Can you work these out from the model? Positions are in its coordinate system, mm. A direction names the side the tool comes from. Give positions to 0.01 mm unless a question says otherwise; leave off trailing zeros. Loops run counter-clockwise (first coordinate to the right, second up) from the corner with the lowest first, then second, coordinate; pieces in that order, holes last. Notation, with made-up numbers: M 41.25,70.5 L 71.25,70.5 A20 cw 71.25,93.5 Z; hole C 50.5,-27 d7. An arc over 180 degrees is marked long. One line per item, written item: value. Start each with the question number.
Solid Edge part; units mm, degrees
sketch "Sketch1" plane through (0, 0, 0) normal (0, 0, 1) x (1, 0, 0)
  circle A0 centre (-86, 0) radius 8
  circle A1 centre (-43, -74.4782) radius 8
  circle A2 centre (43, -74.4782) radius 8
  circle A3 centre (86, 0) radius 8
  circle A4 centre (43, 74.4782) radius 8
  circle A5 centre (-43, 74.4782) radius 8
  circle A6 centre (0, 0) radius 101.5
extrude "Protrusion1" add sketch "Sketch1" along normal blind 19
sketch "Sketch2" plane through (0, 0, 19) normal (0, 0, 1) x (0, 1, 0)
  circle A0 centre (0, 0) radius 32
  circle A1 centre (0, 0) radius 16
extrude "ExtrudedProtrusion_4" add sketch "Sketch2" along normal blind 51
sketch "Sketch3" plane through (0, 0, 0) normal (1, 0, 0) x (0, 1, 0)
  line L0 (-101.5, 19) -> (-32, 70)
  line L1 (-32, 70) -> (-30, 70)
  line L2 (-30, 70) -> (-30, 19)
  line L3 (-30, 19) -> (-101.5, 19)
extrude "ExtrudedCutout_5" cut sketch "Sketch3" along normal mid plane 16
sketch "Sketch4" plane through (0, 0, 0) normal (1, 0, 0) x (0, 1, 0)
  line L0 (-101.5, 19) -> (-32, 70)
  line L1 (-32, 70) -> (-30, 70)
  line L2 (-30, 70) -> (-30, 19)
  line L3 (-30, 19) -> (-101.5, 19)
extrude "ExtrudedProtrusion_9" add sketch "Sketch4" along normal mid plane 16
pattern_circular "Pattern1" count 3 over 360 about axis through (0, 0, 70) along (0, 0, 1) of "ExtrudedProtrusion_9"
Q1. If we section it at B-B, the plane x = -43: Write out the boundary of the cut face in (y, z).
Q2. For P1, Ø21, axis at x = -86, y = 0, coming from the +Z side; P2, Ø5, axis at x = 6, y = -47, coming from the -Z side; P3, Ø14.5, axis at x = 43, y = -74.48, coming from the +Z side; P4, Ø10, axis at x = -28, z = 44, coming from the +Y side, each with a flat end and sliding along its axis, tell me the tip position at first contact or that it passes through.
Q3. If we section it at C-C, the plane z = 39: Write out the boundary of the cut face in (x, y).
Q4. If we mould it in two halves opening along X, with no side actions, what happens to faces 1 (the face through (-48.9, -79.88, 9.37)), 2 (the face through (96.813, -30.488, 9.367)), 3 (the face through (-8, -51, 34))? For each: released by +X, released by -X, zero draft, split by the parting line, or undercut.
Q5. If we section it at A-A, the plane y = 0: Write out the boundary of the cut face in (x, z), plus the area to 3 significant figures.
Q6. If we section it at D-D, the plane y = -88.5: Write out the boundary of the cut face in (x, z), plus the area to 3 significant figures.
Q7. Which directions (+Z, -Z, +X, -X, +Y, -Y) give clear straight access to the entire face, cutting with the end or side of a thin tool? Please do faces 4 (the face through (0, 0, 19)), 5 (the face through (54, -28, 19)), 6 (the face through (-40.22, 32.46, 33.52)), 7 (the face through (27.89, -15.69, 44.14)), 8 (the face through (-0.11, -67.24, 44.14)).
Q8. I need wall thicknesses on line 1 along Y through (x, z) = (-43, 9); line 2 along Y through (x, z) = (44, 12); line 3 along X through (y, z) = (28.5, 59). Which ranges of each line are inside material? Lowest first, please.
Response:
1. outline: M -91.94,0 L -82.48,0 L -82.48,19 L -91.94,19 Z; M -66.48,0 L 66.48,0 L 66.48,19 L 34.06,19 L 34.06,53.66 L 15.59,60.44 L 15.59,19 L -66.48,19 Z; M 82.48,0 L 91.94,0 L 91.94,19 L 82.48,19 Z
2. P1: z = 19
2. P2: z = 0
2. P3: through
2. P4: y = 28.29
3. outline: M -68.3,30.19 L -30.83,8.56 A32 ccw -8,-30.98 L -8,-74.25 L 8,-74.25 L 8,-30.98 A32 ccw 30.83,8.56 L 68.3,30.19 L 60.3,44.05 L 22.83,22.42 A32 ccw -22.83,22.42 L -60.3,44.05 Z; hole C 0,0 d32
4. face 1: undercut
4. face 2: split by the parting line
4. face 3: released by -X
5. outline: M -101.5,0 L -94,0 L -94,19 L -101.5,19 Z; M -78,0 L 78,0 L 78,19 L 32,19 L 32,70 L 16,70 L 16,19 L -16,19 L -16,70 L -32,70 L -32,19 L -78,19 Z; M 94,0 L 101.5,0 L 101.5,19 L 94,19 Z
5. area: 4,880 mm^2
6. outline: M -49.7,0 L 49.7,0 L 49.7,19 L 8,19 L 8,28.54 L -8,28.54 L -8,19 L -49.7,19 Z
6. area: 2,040 mm^2
7. face 4: +Z
7. face 5: +Z, +X, -Y
7. face 6: +Z, +Y
7. face 7: +Z, +X
7. face 8: +Z, +X, -X, -Y
8. line 1: -91.94 to -82.48, -66.48 to 66.48, 82.48 to 91.94
8. line 2: -91.47 to -82.42, -66.54 to 66.54, 82.42 to 91.47
8. line 3: -37.81 to -33.36, -14.55 to 14.55, 33.36 to 37.81
